Model file for the job. Use its own axes, mm. A direction names the side the tool comes from. Round coordinates to 2 decimals unless told otherwise and drop trailing zeros. Write each loop counter-clockwise with the first axis right and the second up, starting at its lowest first coordinate (ties: lowest second). Pieces come first, ordered by that corner, then holes. Notation, with made-up numbers: (-26, 55) - (13, 55) arc R9 ccw to (13, 59) - close; hole circle Ø11 at (1.25, 13.5). An arc over 180 degrees is marked (long way). One line per item, written item: value.
from build123d import *

# Parameters (mm, degrees)
SKETCH7_R           = 5
BOSS_EXTRUDE1_DEPTH = 2.5
FILLET3_R           = 15


with BuildPart() as part:
    # Sketch4 → Revolve1 (revolve)
    with BuildSketch(Plane.XY, mode=Mode.PRIVATE) as revolve1_sk:
        Polygon((5, 5), (5, -5), (6, -5), (6, -25), (15, -25), (15, 25), (6, 25), (6, 5), align=None)
    revolve(revolve1_sk.sketch.rotate(Axis((0, 25, 0), (0, -1, 0)), 90), axis=Axis((0, 25, 0), (0, -1, 0)))

    # Sketch7 → Boss-Extrude1 (add, symmetric)
    with BuildSketch(Plane(origin=(0, 0, 0), x_dir=(1, 0, 0), z_dir=(0, 1, 0))):
        with BuildLine():
            Line((-15, 129.126781955), (-15, 12.5))
            Line((-15, 12.5), (-8.291561976, 12.5))
            ThreePointArc((-8.291561976, 12.5), (-4.330127019, 14.361406616), (0, 15))
            ThreePointArc((0, 15), (10.606601718, 10.606601718), (15, 0))
            Line((15, 0), (15, 99.126781955))
            Line((15, 99.126781955), (37.082039325, 99.126781955))
            ThreePointArc((37.082039325, 99.126781955), (52.082039325, 114.126781955), (37.082039325, 129.126781955))
            Line((37.082039325, 129.126781955), (-15, 129.126781955))
        make_face()
        with Locations(Location((37.082039325, 114.126781955, 0), (0, 0, 270))):
            Circle(SKETCH7_R, mode=Mode.SUBTRACT)
    extrude(amount=BOSS_EXTRUDE1_DEPTH, both=True)

    # Fillet3
    fillet3_edges = [part.edges().sort_by_distance(p)[0] for p in [
        (15, 0, -99.126781955),
        (-15, 0, -129.126781955),
    ]]
    fillet(fillet3_edges, radius=FILLET3_R)


solid = part.part
1. Wall check: probe 1 along X at (y, z) = (-2.25, 0); probe 2 along X at (y, z) = (-13.75, 0); probe 3 along Z at (x, y) = (0.5, 16.5). Give the ranges that are in metal, low to high. Write a range as [from, to].
Report:
probe 1: [-15, -5], [5, 15]
probe 2: [-15, -6], [6, 15]
probe 3: [-14.99, -5.98], [5.98, 14.99]
2. Band-saw the part on A-A on y = 19. Write the cut outline in (x, z).
Report:
outline: circle Ø30 at (0, 0); hole circle Ø12 at (0, 0)
3. Band-saw the part on D-D on x = 26.5. Write the cut outline in (y, z), plus the area to 3 significant figures.
Report:
outline: (-2.5, -129.13) - (2.5, -129.13) - (2.5, -98.71) - (-2.5, -98.71) - close
area: 152 mm²
4. Drop flat-ended pins along their axis: pin 1 (3.5 mm diameter, centred on x = -2.5, z = 2, fed in from -Y); pin 2 (4 mm diameter, centred on y = -0.5, z = -48, fed in from +X); pin 3 (2.5 mm diameter, centred on x = -10.5, y = -1, fed in from +Z); pin 4 (11 mm diameter, centred on x = 0, z = 0, fed in from +Y). Give the stop position or say it passes through.
Report:
pin 1: through
pin 2: x = 15
pin 3: z = 11.81
pin 4: y = 5
5. Band-saw the part on B-B on x = 2.5. Write the cut outline in (y, z), plus the area to 3 significant figures.
Report:
outline: (-25, -14.79) - (-2.5, -14.79) - (-2.5, -129.13) - (2.5, -129.13) - (2.5, -14.79) - (25, -14.79) - (25, -5.45) - (5, -5.45) - (5, -4.33) - (-5, -4.33) - (-5, -5.45) - (-25, -5.45) - close; (-25, 5.45) - (-5, 5.45) - (-5, 4.33) - (5, 4.33) - (5, 5.45) - (25, 5.45) - (25, 14.79) - (-25, 14.79) - close
area: 1,530 mm²
6. Band-saw the part on C-C on z = -11. Write the cut outline in (x, y), plus the area to 3 significant figures.
Report:
outline: (-10.2, -25) - (10.2, -25) - (10.2, -2.5) - (15, -2.5) - (15, 2.5) - (10.2, 2.5) - (10.2, 25) - (-10.2, 25) - close
area: 1,040 mm²
7. Tool access for faces 4 (the face through (-4, -5, 4)), 5 (the face through (-10.72, -0.04, -124.62)), 6 (the face through (33, 0, -99.127)), 7 (the face through (-12.65, 0.35, 8.06)), 8 (the face through (-4, 5, -4)): list every direction of +Z, -Z, +X, -X, +Y, -Y with a clear straight run to the whole face (end or side of a thin tool).
Report:
face 4: -Y
face 5: -Z, -X, +Y, -Y
face 6: +Z, +X, +Y, -Y
face 7: none
face 8: +Y
8. Mould opens along Z. For faces 1 (the face through (19.28, -0.04, -94.62)), 2 (the face through (-1.802, -15.14, 5.723)), 3 (the face through (19, 0, -129.127)) say: released by +Z, released by -Z, zero draft, split by the parting line, or undercut.
Report:
face 1: released by +Z
face 2: undercut
face 3: released by -Z
